Could you check a few things on this model? Use its own coordinates, in mm. A direction names the side the tool comes from. Coordinates: 2 decimals unless noted, no trailing zeros. Loops run counter-clockwise (first coordinate to the right, second up) from the corner with the lowest first, then second, coordinate; pieces in that order, holes last.
from build123d import *

# Parameters (mm, degrees)
F0_R     = 38.1
F0_R_2   = 31.75
F1_DEPTH = 304.8
F2_R     = 25.4
F3_DEPTH = 127


with BuildPart() as f1:
    # F0 (on Front) → F1 (new body, symmetric)
    with BuildSketch(Plane.XZ):
        Circle(F0_R)
        Circle(F0_R_2, mode=Mode.SUBTRACT)
    extrude(amount=F1_DEPTH, both=True)

    # F2 (on Right) → F3 (join, symmetric)
    with BuildSketch(Plane.YZ):
        Circle(F2_R)
    extrude(amount=F3_DEPTH, both=True)


solid = f1.part
(1) Imagine slicing it at C-C, the plane y = 0. Write out the boundary of the cut face in (x, z).
Answers:
outline: (-127, -25.4) - (-28.4, -25.4) arc R38.1 ccw to (28.4, -25.4) - (127, -25.4) - (127, 25.4) - (28.4, 25.4) arc R38.1 ccw to (-28.4, 25.4) - (-127, 25.4) - close; hole (-19.05, -25.4) arc R31.75 ccw to (19.05, -25.4) - close; hole (-19.05, 25.4) - (19.05, 25.4) arc R31.75 ccw to start
(2) For pin 1 (5 mm diameter, centred on x = -88, z = -0.5, fed in from +Y); pin 2 (6 mm diameter, centred on y = 78, z = 21, fed in from -X); pin 3 (3 mm diameter, centred on x = -95.5, z = -12, fed in from +Y), each with a flat end and sliding along its axis, tell me the tip position at first contact or that it passes through.
Answers:
pin 1: stops at y = 25.4
pin 2: stops at x = -33.58
pin 3: stops at y = 23.13
(3) We'd pull the mould along X, two halves only. Please class faces 4 (the face through (-127, 0, 0)), 5 (the face through (-77.009, 24.227, 7.629)), 6 (the face through (127, 0, 0)), 7 (the face through (0.444, 24.227, 7.629)): +X half, -X half, draft (parallel to the pull), parting line (faces both ways), or undercut.
Answers:
face 4: -X half
face 5: draft
face 6: +X half
face 7: undercut
(4) I need wall thicknesses on probe 1 along X at (y, z) = (91, 0); probe 2 along X at (y, z) = (62, -2). Which ranges of each line are inside material? Lowest first, please.
Answers:
probe 1: x = -38.1 to -31.75, 31.75 to 38.1
probe 2: x = -38.05 to -31.69, 31.69 to 38.05
(5) Which directions (+Z, -Z, +X, -X, +Y, -Y) give clear straight access to the entire face, cutting with the end or side of a thin tool? Please do faces 1 (the face through (-4.96, -4.267, 37.776)), 2 (the face through (-9, 304.8, 31)), 3 (the face through (78.389, -3.307, 25.184)).
Answers:
face 1: none
face 2: +Z, -Z, +X, -X, +Y
face 3: +X
(6) Imagine slicing it at A-A, the plane x = 0. Write out the boundary of the cut face in (y, z).
Answers:
outline: (-304.8, -38.1) - (304.8, -38.1) - (304.8, -31.75) - (-304.8, -31.75) - close; (-304.8, 31.75) - (304.8, 31.75) - (304.8, 38.1) - (-304.8, 38.1) - close; circle Ø50.8 at (0, 0)
(7) Imagine slicing it at B-B, the plane z = 0. Write out the boundary of the cut face in (x, y), and give its area (3 significant figures).
Answers:
outline: (-127, -25.4) - (-38.1, -25.4) - (-38.1, -304.8) - (-31.75, -304.8) - (-31.75, -25.4) - (31.75, -25.4) - (31.75, -304.8) - (38.1, -304.8) - (38.1, -25.4) - (127, -25.4) - (127, 25.4) - (38.1, 25.4) - (38.1, 304.8) - (31.75, 304.8) - (31.75, 25.4) - (-31.75, 25.4) - (-31.75, 304.8) - (-38.1, 304.8) - (-38.1, 25.4) - (-127, 25.4) - close
area: 20,000 mm2
(8) Imagine slicing it at D-D, the plane y = 79. Write out the boundary of the cut face in (x, z), and give its area (3 significant figures).
Answers:
outline: circle Ø76.2 at (0, 0); hole circle Ø63.5 at (0, 0)
area: 1,390 mm2
